CAD build for the part. Positions are in the model's coordinates, mm. A direction names the side the tool comes from. Give positions to 0.01 mm unless a question says otherwise; leave off trailing zeros. Order: outer loops, then holes, each group sorted by start corner. A loop starts at its lowest first (then second) coordinate and runs counter-clockwise, first axis right, second up. Notation, with made-up numbers: M -39.5,44.5 L 19.5,44.5 A8 cw 19.5,49.5 Z; hole C -37.5,20.25 d1. An arc over 180 degrees is marked long. Put each result on its own line as item: value. Start each with the question number.
1) Cut at B-B (x = 0). Write the cut outline in (y, z) (3 decimals), and give its area (3 significant figures).
2) Drill centre lines: line 1 (X direction, y = -7, z = -22); line 2 (Z direction, x = -8, y = -2.75); line 3 (X direction, y = -4.5, z = -9.5). Where is each one in solid material? Low to high. Write a range as [from, to].
3) Cut at A-A (z = -13). Write the cut outline in (x, y) (3 decimals), and give its area (3 significant figures).
4) Cut at C-C (z = 13.3). Write the cut outline in (x, y) (3 decimals), and give its area (3 significant figures).
5) Two-plate mould, pull along Z, no slides. Class faces 1 (the face through (17, -10.775, 0)), 2 (the face through (0, -3, 25)), 3 (the face through (17.55, -9.3, -17.3)), 4 (the face through (-16.384, -6.438, -15.998)): released by +Z, released by -Z, zero draft, split by the parting line, or undercut.
6) Tool access for faces 5 (the face through (-18, -9, -13.7)), 6 (the face through (2.872, -2.421, 16.432)), 7 (the face through (-15.25, -8, 0)), 8 (the face through (18, -9, 15.3)): list every direction of +Z, -Z, +X, -X, +Y, -Y with a clear straight run to the whole face (end or side of a thin tool).
7) Cut at D-D (x = -7.5). Write the cut outline in (y, z) (3 decimals).
8) Pin check, flat tip, straight feed: pin 1 (4 mm diameter, centred on y = -7.975, z = 17.8, fed in from +X). Stop position of the tip, or through.
```python
from build123d import *

# Parameters (mm, degrees)
SKETCH1_W              = 50
SKETCH1_H              = 10.775
BOSS_EXTRUDE1_DEPTH    = 19.05
SKETCH2_W              = 30.5
SKETCH2_H              = 6
CUT_EXTRUDE1_DEPTH     = 55.580244824
SKETCH3_R              = 4.25
CUT_EXTRUDE2_DEPTH     = 32.998476526
M2_CLEARANCE_HOLE1_D   = 2.6
M2_5_CLEARANCE_HOLE1_D = 3.1
CUT_EXTRUDE3_DEPTH     = 1.5
CUT_EXTRUDE4_START     = -36.6
CUT_EXTRUDE4_DEPTH     = 1.5
FILLET1_R              = 1
FILLET2_R              = 3
SKETCH9_W              = 7
SKETCH9_H              = 12
CUT_EXTRUDE5_DEPTH     = 34.226542477


with BuildPart() as part:
    # Sketch1 → Boss-Extrude1 (new, symmetric)
    with BuildSketch(Plane(origin=(0, 0, 0), x_dir=(0, 0, -1), z_dir=(1, 0, 0))):
        with Locations((0, -5.3875)):
            Rectangle(SKETCH1_W, SKETCH1_H)
    extrude(amount=BOSS_EXTRUDE1_DEPTH, both=True)

    # Sketch2 → Cut-Extrude1 (cut, through all)
    with BuildSketch(Plane.XY.offset(25)):
        with Locations((0, -7.775)):
            Rectangle(SKETCH2_W, SKETCH2_H)
    extrude(amount=-CUT_EXTRUDE1_DEPTH, mode=Mode.SUBTRACT)

    # Sketch3 → Cut-Extrude2 (cut, through all)
    with BuildSketch(Plane.XZ.offset(4.775)):
        with Locations(Location((0, 13.3, 0), (0, 0, 270))):
            Circle(SKETCH3_R)
    extrude(amount=-CUT_EXTRUDE2_DEPTH, mode=Mode.SUBTRACT)

    # M2 Clearance Hole1 (through all)
    with Locations(Plane(origin=(0, -4.775, 0), x_dir=(-1, 0, 0), z_dir=(0, -1, 0))):
        with Locations((8, -13.3), (0, -21.3), (-8, -13.3), (0, -5.3)):
            Hole(M2_CLEARANCE_HOLE1_D / 2)

    # M2.5 Clearance Hole1 (through all)
    with Locations(Plane.ZY.offset(19.05)):
        with Locations((-16.2, -7.975), (17.8, -7.975)):
            Hole(M2_5_CLEARANCE_HOLE1_D / 2)

    # Sketch8 → Cut-Extrude3 (cut)
    with BuildSketch(Plane(origin=(19.05, 0, 0), x_dir=(0, 0, -1), z_dir=(1, 0, 0))):
        with BuildLine():
            Line((-20.3, -7.975), (-20.3, -10.775))
            Line((-20.3, -10.775), (-15.3, -10.775))
            Line((-15.3, -10.775), (-15.3, -7.975))
            ThreePointArc((-15.3, -7.975), (-17.8, -5.475), (-20.3, -7.975))
        make_face()
        with BuildLine():
            Line((13.7, -7.975), (13.7, -10.775))
            Line((13.7, -10.775), (18.7, -10.775))
            Line((18.7, -10.775), (18.7, -7.975))
            ThreePointArc((18.7, -7.975), (16.2, -5.475), (13.7, -7.975))
        make_face()
    extrude(amount=-CUT_EXTRUDE3_DEPTH, mode=Mode.SUBTRACT)

    # Sketch8<2> → Cut-Extrude4 (cut)
    with BuildSketch(Plane(origin=(19.05, 0, 0), x_dir=(0, 0, -1), z_dir=(1, 0, 0)).offset(CUT_EXTRUDE4_START)):
        with BuildLine():
            Line((-20.3, -7.975), (-20.3, -10.775))
            Line((-20.3, -10.775), (-15.3, -10.775))
            Line((-15.3, -10.775), (-15.3, -7.975))
            ThreePointArc((-15.3, -7.975), (-17.8, -5.475), (-20.3, -7.975))
        make_face()
        with BuildLine():
            Line((13.7, -7.975), (13.7, -10.775))
            Line((13.7, -10.775), (18.7, -10.775))
            Line((18.7, -10.775), (18.7, -7.975))
            ThreePointArc((18.7, -7.975), (16.2, -5.475), (13.7, -7.975))
        make_face()
    extrude(amount=-CUT_EXTRUDE4_DEPTH, mode=Mode.SUBTRACT)

    # Fillet1
    fillet1_edges = [part.edges().sort_by_distance(p)[0] for p in [
        (-15.25, -4.775, 0),
        (15.25, -4.775, 0),
    ]]
    fillet(fillet1_edges, radius=FILLET1_R)

    # Fillet2
    fillet2_edges = [part.edges().sort_by_distance(p)[0] for p in [
        (19.05, 0, 0),
        (-19.05, 0, 0),
    ]]
    fillet(fillet2_edges, radius=FILLET2_R)

    # Sketch9 → Cut-Extrude5 (cut, through all)
    with BuildSketch(Plane(origin=(0, 0, 0), x_dir=(1, 0, 0), z_dir=(0, 1, 0))):
        with Locations((0, 10)):
            Rectangle(SKETCH9_W, SKETCH9_H)
    extrude(amount=-CUT_EXTRUDE5_DEPTH, mode=Mode.SUBTRACT)


solid = part.part
```
Solution:
1. outline: M -4.775,-25 L 0,-25 L 0,-16 L -4.775,-16 Z; M -4.775,-4 L 0,-4 L 0,4 L -4.775,4 Z; M -4.775,6.6 L 0,6.6 L 0,9.05 L -4.775,9.05 Z; M -4.775,17.55 L 0,17.55 L 0,20 L -4.775,20 Z; M -4.775,22.6 L 0,22.6 L 0,25 L -4.775,25 Z
1. area: 116 mm²
2. line 1: [-19.05, -15.25], [15.25, 19.05]
2. line 2: [-25, 12], [14.6, 25]
2. line 3: [-19.05, -3.5], [3.5, 19.05]
3. outline: M -19.05,-10.775 L -15.25,-10.775 L -15.25,-5.775 A1 cw -14.25,-4.775 L -3.5,-4.775 L -3.5,0 L -16.05,0 A3 ccw -19.05,-3 Z; M 3.5,-4.775 L 14.25,-4.775 A1 cw 15.25,-5.775 L 15.25,-10.775 L 19.05,-10.775 L 19.05,-3 A3 ccw 16.05,0 L 3.5,0 Z
3. area: 191 mm²
4. outline: M -19.05,-10.775 L -15.25,-10.775 L -15.25,-5.775 A1 cw -14.25,-4.775 L -9.3,-4.775 L -9.3,0 L -16.05,0 A3 ccw -19.05,-3 Z; M -6.7,-4.775 L -4.25,-4.775 L -4.25,0 L -6.7,0 Z; M 4.25,-4.775 L 6.7,-4.775 L 6.7,0 L 4.25,0 Z; M 9.3,-4.775 L 14.25,-4.775 A1 cw 15.25,-5.775 L 15.25,-10.775 L 19.05,-10.775 L 19.05,-3 A3 ccw 16.05,0 L 9.3,0 Z
4. area: 159 mm²
5. face 1: zero draft
5. face 2: released by +Z
5. face 3: undercut
5. face 4: undercut
6. face 5: -X, -Y
6. face 6: +Y, -Y
6. face 7: +Z, -Z, -Y
6. face 8: +X, -Y
7. outline: M -4.775,-25 L 0,-25 L 0,12.1 L -4.775,12.1 Z; M -4.775,14.5 L 0,14.5 L 0,25 L -4.775,25 Z
8. pin 1: x = 17.55
